```python
from build123d import *

# Parameters (mm, degrees)
SKETCH1_W            = 228.6
SKETCH1_H            = 457.2
BOSS_EXTRUDE1_DEPTH  = 12.7
SKETCH2_W            = 12.7
SKETCH2_H            = 101.6
BOSS_EXTRUDE2_DEPTH  = 12.7
SKETCH3_W            = 101.6
SKETCH3_H            = 457.2
BOSS_EXTRUDE3_DEPTH  = 12.7
FILLET1_R            = 12.7
FILLET1_OF_MIRROR1_R = 12.7
SKETCH4_R            = 6.35
CUT_EXTRUDE1_DEPTH   = 823.269834057
FILLET2_R            = 50.8
FILLET3_R            = 50.8
FILLET4_R            = 50.8
FILLET5_R            = 50.8
SKETCH5_R            = 12.7
CUT_EXTRUDE2_DEPTH   = 687.387711137
SKETCH6_R            = 12.7
CUT_EXTRUDE3_DEPTH   = 687.387711137


with BuildPart() as part:
    # Sketch1 → Boss-Extrude1 (new body)
    with BuildSketch(Plane(origin=(0, 0, 0), x_dir=(1, 0, 0), z_dir=(0, 1, 0))):
        with Locations((114.3, 228.6)):
            Rectangle(SKETCH1_W, SKETCH1_H)
    boss_extrude1 = extrude(amount=BOSS_EXTRUDE1_DEPTH)

    # Sketch2 → Boss-Extrude2 (add)
    with BuildSketch(Plane(origin=(0, 12.7, 0), x_dir=(1, 0, 0), z_dir=(0, 1, 0))):
        with Locations((234.95, 228.6)):
            Rectangle(SKETCH2_W, SKETCH2_H)
    boss_extrude2 = extrude(amount=-BOSS_EXTRUDE2_DEPTH)

    # Sketch3 → Boss-Extrude3 (add)
    with BuildSketch(Plane(origin=(241.3, 0, 0), x_dir=(0, 0, -1), z_dir=(1, 0, 0))):
        with Locations((228.6, 228.6)):
            Rectangle(SKETCH3_W, SKETCH3_H)
    boss_extrude3 = extrude(amount=BOSS_EXTRUDE3_DEPTH)

    # Fillet1
    fillet1_edges = [part.edges().sort_by_distance(p)[0] for p in [
        (241.3, 12.7, -228.6),
    ]]
    fillet(fillet1_edges, radius=FILLET1_R)

    # Mirror1: Boss-Extrude1, Boss-Extrude2, Boss-Extrude3 across plane
    add(boss_extrude1.mirror(Plane(origin=(0, 12.7, 0), x_dir=(0, 0, 1), z_dir=(1, 0, 0))))
    add(boss_extrude2.mirror(Plane(origin=(0, 12.7, 0), x_dir=(0, 0, 1), z_dir=(1, 0, 0))))
    add(boss_extrude3.mirror(Plane(origin=(0, 12.7, 0), x_dir=(0, 0, 1), z_dir=(1, 0, 0))))

    # Fillet1 of Mirror1
    fillet1_of_mirror1_edges = [part.edges().sort_by_distance(p)[0] for p in [
        (-241.3, 12.7, -228.6),
    ]]
    fillet(fillet1_of_mirror1_edges, radius=FILLET1_OF_MIRROR1_R)

    # Sketch4 → Cut-Extrude1 (cut, through all)
    with BuildSketch(Plane.ZY.offset(254)):
        with Locations((-228.6, 406.4)):
            Circle(SKETCH4_R)
    extrude(amount=-CUT_EXTRUDE1_DEPTH, mode=Mode.SUBTRACT)

    # Fillet2
    fillet2_edges = [part.edges().sort_by_distance(p)[0] for p in [
        (-247.65, 457.2, -177.8),
    ]]
    fillet(fillet2_edges, radius=FILLET2_R)

    # Fillet3
    fillet3_edges = [part.edges().sort_by_distance(p)[0] for p in [
        (-247.65, 457.2, -279.4),
    ]]
    fillet(fillet3_edges, radius=FILLET3_R - 0.0001)  # a hair under: the kernel refuses the full size

    # Fillet4
    fillet4_edges = [part.edges().sort_by_distance(p)[0] for p in [
        (247.65, 457.2, -177.8),
    ]]
    fillet(fillet4_edges, radius=FILLET4_R)

    # Fillet5
    fillet5_edges = [part.edges().sort_by_distance(p)[0] for p in [
        (247.65, 457.2, -279.4),
    ]]
    fillet(fillet5_edges, radius=FILLET5_R - 0.0001)  # a hair under: the kernel refuses the full size

    # Sketch5 → Cut-Extrude2 (cut, through all)
    with BuildSketch(Plane(origin=(0, 12.7, 0), x_dir=(1, 0, 0), z_dir=(0, 1, 0))):
        with Locations(Location((-177.8, 406.4, 0), (0, 0, 270))):
            Circle(SKETCH5_R)
    extrude(amount=-CUT_EXTRUDE2_DEPTH, mode=Mode.SUBTRACT)

    # Sketch6 → Cut-Extrude3 (cut, through all)
    with BuildSketch(Plane(origin=(0, 12.7, 0), x_dir=(1, 0, 0), z_dir=(0, 1, 0))):
        with Locations(Location((177.8, 406.4, 0), (0, 0, 270))):
            Circle(SKETCH6_R)
        with Locations(Location((-177.8, 50.8, 0), (0, 0, 270))):
            Circle(SKETCH6_R)
        with Locations(Location((177.8, 50.8, 0), (0, 0, 270))):
            Circle(SKETCH6_R)
    extrude(amount=-CUT_EXTRUDE3_DEPTH, mode=Mode.SUBTRACT)


solid = part.part
```
Model file for the job. Use its own axes, mm. A direction names the side the tool comes from. Coordinates: 2 decimals unless noted, no trailing zeros. Write each loop counter-clockwise with the first axis right and the second up, starting at its lowest first coordinate (ties: lowest second). Pieces come first, ordered by that corner, then holes. Notation, with made-up numbers: (9.5, 60) - (23.5, 60) arc R20 ccw to (23.5, 89) - close; hole circle Ø4 at (21, 60.5). An arc over 180 degrees is marked (long way). One line per item, written item: value. Start each with the question number.
1. Slice it at C-C (x = -177.8). Write the cut outline in (y, z), plus the area to 3 significant figures.
2. Slice it at B-B (y = 253). Write the cut outline in (x, z), plus the area to 3 significant figures.
3. Mould opens along X. For faces 1 (the flat face through (-254, 232, -228)), 2 (the flat face through (247, 200, -177.8)), 3 (the flat face through (241.3, 244, -228)) say: released by +X, released by -X, zero draft, split by the parting line, or undercut.
4. Probe line 1 (X direction, y = 8.5, z = -406.4); line 2 (Y direction, x = 244.25, z = -228.6); line 3 (Z direction, x = 246.5, y = 406.4). List the from-to ranges inside material, lowest first. Write a range as from..to.
5. Slice it at D-D (z = -246). Write the cut outline in (x, y).
6. Tool access for faces 4 (the flat face through (-228.6, 6, -367)), 5 (the flat face through (-228.6, 6, -88)), 6 (the flat face through (228.6, 6, -367)), 7 (the flat face through (-241.3, 244, -228)): list every direction of +Z, -Z, +X, -X, +Y, -Y with a clear straight run to the whole face (end or side of a thin tool).
7. Slice it at A-A (z = -50.8). Write the cut outline in (x, y).
8. Flat gauge pins, fed straight in: pin 1 (20.5 mm diameter, centred on x = 177.8, z = -50.8, fed in from +Y); pin 2 (2 mm diameter, centred on x = 133.5, z = -214, fed in from +Y); pin 3 (6.5 mm diameter, centred on y = 6, z = -101, fed in from +X); pin 4 (6.5 mm diameter, centred on y = 8.5, z = -353, fed in from -X). Where does each tip first touch, or does it go through?
Answers below:
1. outline: (0, -457.2) - (12.7, -457.2) - (12.7, -419.1) - (0, -419.1) - close; (0, -393.7) - (12.7, -393.7) - (12.7, -63.5) - (0, -63.5) - close; (0, -38.1) - (12.7, -38.1) - (12.7, 0) - (0, 0) - close
1. area: 5,160 mm^2
2. outline: (-254, -279.4) - (-241.3, -279.4) - (-241.3, -177.8) - (-254, -177.8) - close; (241.3, -279.4) - (254, -279.4) - (254, -177.8) - (241.3, -177.8) - close
2. area: 2,580 mm^2
3. face 1: released by -X
3. face 2: zero draft
3. face 3: undercut
4. line 1: x = -228.6..-190.5, -165.1..165.1, 190.5..228.6
4. line 2: y = 0..400.05, 412.75..457.2
4. line 3: z = -279.4..-234.95, -222.25..-177.8
5. outline: (-254, 0) - (254, 0) - (254, 454.13) - (241.3, 454.13) - (241.3, 25.4) arc R12.7 cw to (228.6, 12.7) - (-228.6, 12.7) arc R12.7 cw to (-241.3, 25.4) - (-241.3, 454.13) - (-254, 454.13) - close
6. face 4: -Z, -X, +Y, -Y
6. face 5: +Z, -X, +Y, -Y
6. face 6: -Z, +X, +Y, -Y
6. face 7: +Z, -Z, +Y
7. outline: (-228.6, 0) - (-190.5, 0) - (-190.5, 12.7) - (-228.6, 12.7) - close; (-165.1, 0) - (165.1, 0) - (165.1, 12.7) - (-165.1, 12.7) - close; (190.5, 0) - (228.6, 0) - (228.6, 12.7) - (190.5, 12.7) - close
8. pin 1: passes through
8. pin 2: stops at y = 12.7
8. pin 3: stops at x = 228.6
8. pin 4: stops at x = -228.6
